Read the model definition and answer for the solid it produces. Units are mm, in the model's axes. A direction names the side the tool comes from. Coordinates: 2 decimals unless noted, no trailing zeros. Order: outer loops, then holes, each group sorted by start corner. A loop starts at its lowest first (then second) coordinate and runs counter-clockwise, first axis right, second up. Notation, with made-up numbers: (3, 70) -> (28, 70) arc R18 ccw to (28, 81) -> close; hole circle Ø4 at (45.5, -14.75). An arc over 180 degrees is marked (long way). Use CSV: the item, a comma, the result in double quotes.
```python
from build123d import *

# Parameters (mm, degrees)
SKETCH_1_W          = 66
SKETCH_1_H          = 66
SKETCH_1_W_2        = 42
SKETCH_1_H_2        = 42
EXTRUDE_1_DEPTH     = 110
SKETCH_2_W          = 42
SKETCH_2_H          = 42
CUT_EXTRUDE_1_DEPTH = 76
SKETCH_3_R          = 18
CUT_EXTRUDE_2_DEPTH = 28
SKETCH_4_R          = 11
CUT_EXTRUDE_3_DEPTH = 2
SKETCH_5_R          = 1.5
SKETCH_5_R_2        = 2
CUT_EXTRUDE_4_DEPTH = 120.490585403
CHAMFER_1_SIZE      = 6
CUT_EXTRUDE_5_REACH = 134.458
SKETCH_6_W          = 16
SKETCH_6_H          = 25
CUT_EXTRUDE_6_REACH = 134.458
SKETCH_7_W          = 25
SKETCH_7_H          = 10


with BuildPart() as part:
    # 草图1 → 凸台-拉伸1 (new body)
    # profile 1 of 2: a face of its own
    with BuildSketch(Plane(origin=(0, 0, 0), x_dir=(1, 0, 0), z_dir=(0, 1, 0))):
        Rectangle(SKETCH_1_W, SKETCH_1_H)
        Rectangle(SKETCH_1_W_2, SKETCH_1_H_2, mode=Mode.SUBTRACT)
    # profile 2 of 2: a face of its own
    with BuildSketch(Plane(origin=(0, 0, 0), x_dir=(1, 0, 0), z_dir=(0, 1, 0))):
        Rectangle(SKETCH_1_W_2, SKETCH_1_H_2)
    extrude(amount=EXTRUDE_1_DEPTH)

    # 草图2 → 切除-拉伸1 (cut)
    with BuildSketch(Plane.XZ):
        Rectangle(SKETCH_2_W, SKETCH_2_H)
    extrude(amount=-CUT_EXTRUDE_1_DEPTH, mode=Mode.SUBTRACT)

    # 草图3 → 切除-拉伸2 (cut)
    with BuildSketch(Plane.XZ.offset(-76)):
        with Locations(Location((0, 0, 0), (0, 0, 270))):
            Circle(SKETCH_3_R)
    extrude(amount=-CUT_EXTRUDE_2_DEPTH, mode=Mode.SUBTRACT)

    # 草图4 → 切除-拉伸3 (cut)
    with BuildSketch(Plane.XZ.offset(-104)):
        with Locations(Location((0, 0, 0), (0, 0, 270))):
            Circle(SKETCH_4_R)
    extrude(amount=-CUT_EXTRUDE_3_DEPTH, mode=Mode.SUBTRACT)

    # 草图5 → 切除-拉伸4 (cut, through all)
    with BuildSketch(Plane(origin=(0, 110, 0), x_dir=(1, 0, 0), z_dir=(0, 1, 0))):
        with Locations(Location((-9.899494937, 9.899494937, 0), (0, 0, 270))):
            Circle(SKETCH_5_R)
        with Locations(Location((9.899494937, 9.899494937, 0), (0, 0, 270))):
            Circle(SKETCH_5_R)
        with Locations(Location((9.899494937, -9.899494937, 0), (0, 0, 270))):
            Circle(SKETCH_5_R)
        with Locations(Location((-9.899494937, -9.899494937, 0), (0, 0, 270))):
            Circle(SKETCH_5_R)
        with Locations(Location((-27, 27, 0), (0, 0, 270))):
            Circle(SKETCH_5_R_2)
        with Locations(Location((27, 27, 0), (0, 0, 270))):
            Circle(SKETCH_5_R_2)
        with Locations(Location((-27, -27, 0), (0, 0, 270))):
            Circle(SKETCH_5_R_2)
        with Locations(Location((27, -27, 0), (0, 0, 270))):
            Circle(SKETCH_5_R_2)
    extrude(amount=-CUT_EXTRUDE_4_DEPTH, mode=Mode.SUBTRACT)

    # 倒角1
    chamfer_1_edges = [part.edges().sort_by_distance(p)[0] for p in [
        (21, 38, -21),
        (-21, 38, -21),
        (-21, 38, 21),
        (21, 38, 21),
    ]]
    chamfer(chamfer_1_edges, length=CHAMFER_1_SIZE)

    # 草图6 → 切除-拉伸5 (cut, up to next)
    with BuildSketch(Plane(origin=(0, 0, -33), x_dir=(-1, 0, 0), z_dir=(0, 0, -1)), mode=Mode.PRIVATE) as cut_extrude_5_sk1:
        with Locations((0, 12.5)):
            Rectangle(SKETCH_6_W, SKETCH_6_H)
    cut_extrude_5_tool1 = extrude(cut_extrude_5_sk1.sketch, amount=-CUT_EXTRUDE_5_REACH, mode=Mode.PRIVATE) & part.part
    add(cut_extrude_5_tool1.solids().sort_by_distance((0, 12.5, -33))[0], mode=Mode.SUBTRACT)

    # 草图7 → 切除-拉伸6 (cut, up to next)
    with BuildSketch(Plane.ZY.offset(33), mode=Mode.PRIVATE) as cut_extrude_6_sk1:
        with Locations((0, 5)):
            Rectangle(SKETCH_7_W, SKETCH_7_H)
    cut_extrude_6_tool1 = extrude(cut_extrude_6_sk1.sketch, amount=-CUT_EXTRUDE_6_REACH, mode=Mode.PRIVATE) & part.part
    add(cut_extrude_6_tool1.solids().sort_by_distance((-33, 5, 0))[0], mode=Mode.SUBTRACT)


solid = part.part
```
Item 1: The mould has two halves that part along Z. Classify faces 1 (the flat face through (0, 54, 33)), 2 (the cylindrical face through (25.226, 55.77, 27.923)), 3 (the flat face through (0, 110, 0)): +Z half, -Z half, draft (parallel to the pull), parting line (faces both ways), or undercut.
Return value:
face 1,"+Z half"
face 2,"undercut"
face 3,"draft"
Item 2: Find section B-B, the plane y = 100.5. Give the vertices of the cut face in (x, z).
Return value:
outline,"(-33, -33) -> (33, -33) -> (33, 33) -> (-33, 33) -> close; hole circle Ø4 at (-27, -27); hole circle Ø4 at (-27, 27); hole circle Ø36 at (0, 0); hole circle Ø4 at (27, -27); hole circle Ø4 at (27, 27)"
Item 3: A tool of negligible diameter and unlimited length cuts with its end or side. For faces 4 (the flat face through (-27, 10, 0)), 5 (the cylindrical face through (-28.774, 55.77, 27.923)), 6 (the cylindrical face through (5.407, 89.804, -17.169)), 7 (the flat face through (-33, 54, 0)), 8 (the flat face through (-8, 12, -27)), from which of +Z, -Z, +X, -X, +Y, -Y can it reach the whole face along a straight path? Write none if from no direction.
Return value:
face 4,"-X, -Y"
face 5,"+Y, -Y"
face 6,"-Y"
face 7,"+Z, -Z, -X, +Y, -Y"
face 8,"-Z, -Y"
Item 4: Straight lines are drawn through the part: line 1 along X through (y, z) = (71, -27); line 2 along X through (y, z) = (27.5, 1.5); line 3 along X through (y, z) = (65.5, 28.5). For each, find the intervals that lie inside material, in ascending order.
Return value:
line 1,"x = -33 to -29, -25 to 25, 29 to 33"
line 2,"x = -33 to -21, 21 to 33"
line 3,"x = -33 to -28.32, -25.68 to 25.68, 28.32 to 33"
Item 5: Each of these flat-tipped pins is pushed along its axis until it touches: P1, Ø24, axis at x = 5, z = -4.5, coming from the -Y side; P2, Ø5, axis at x = 27, z = 27, coming from the -Y side; P3, Ø5, axis at x = -9.9, z = -9.9, coming from the -Y side; P4, Ø2, axis at x = 4, y = 16.5, coming from the -Z side. Where does it stop, or does it pass through?
Return value:
P1,"stops at y = 76"
P2,"stops at y = 0"
P3,"stops at y = 104"
P4,"stops at z = 21"
Item 6: Find section A-A, the plane x = -27. Give the vertices of the cut face in (y, z).
Return value:
outline,"(0, -33) -> (110, -33) -> (110, -29) -> (0, -29) -> close; (0, -25) -> (110, -25) -> (110, 25) -> (0, 25) -> (0, 12.5) -> (10, 12.5) -> (10, -12.5) -> (0, -12.5) -> close; (0, 29) -> (110, 29) -> (110, 33) -> (0, 33) -> close"
Item 7: Find section D-D, the plane z = -22.5. Give the vertices of the cut face in (x, y).
Return value:
outline,"(-33, 0) -> (-8, 0) -> (-8, 25) -> (8, 25) -> (8, 0) -> (33, 0) -> (33, 110) -> (-33, 110) -> close"
Item 8: Find section C-C, the plane z = 27. Give the vertices of the cut face in (x, y), then the cut area to 3 significant figures.
Return value:
outline,"(-33, 0) -> (-29, 0) -> (-29, 110) -> (-33, 110) -> close; (-25, 0) -> (25, 0) -> (25, 110) -> (-25, 110) -> close; (29, 0) -> (33, 0) -> (33, 110) -> (29, 110) -> close"
area,"6,380 mm^2"
